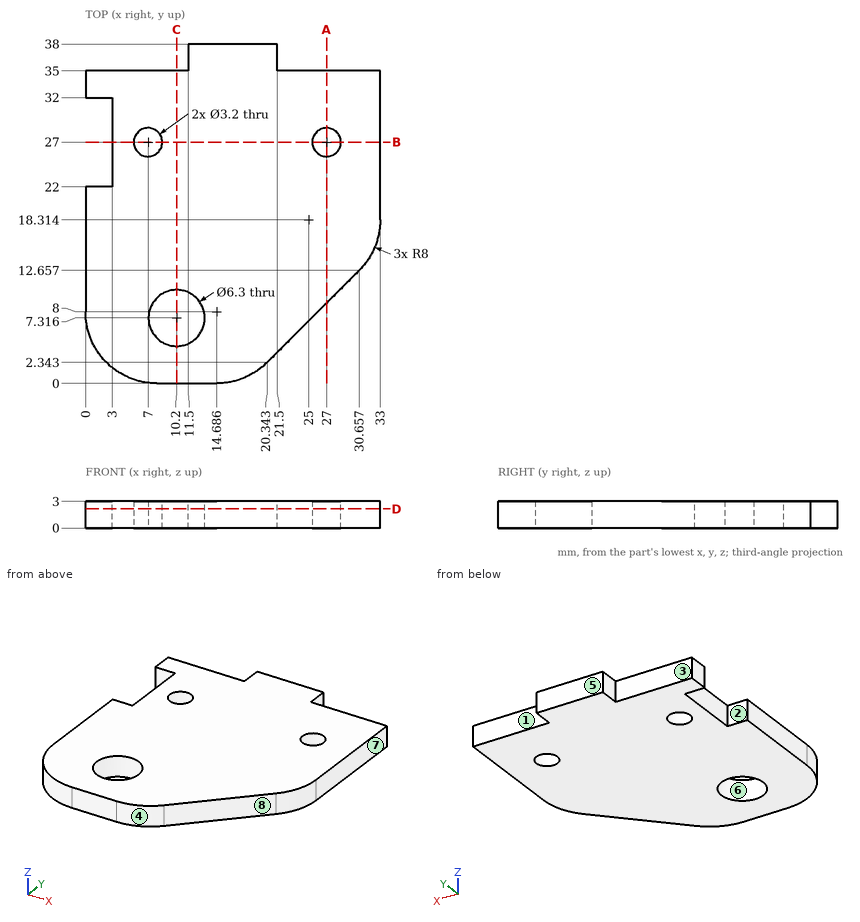
Geometry: see drawing. Coordinates: mm, zero at the bounding-box minimum. A direction names the side the tool comes from. Round coordinates to 2 decimals unless told otherwise and drop trailing zeros. Write each loop counter-clockwise with the first axis right and the second up, starting at its lowest first coordinate (ties: lowest second). Pieces come first, ordered by that corner, then holes.
1) Ray query, L1, parallel to Y at x = 10.2, z = 1.5; L2, parallel to Y at x = 21, z = 0.75; L3, parallel to Y at x = 27, z = 2.5. Return the intervals inside material, ascending.
2) Cut plane B-B (y = 27). Return the cut outline in (x, z), then the cut area to 3 significant figures.
3) Reachability of the marked faces 1, 2, 3 and 4 from +Z, -Z, +X, -X, +Y, -Y: full face, straight path, thin tool, end or side. Return the list, or none.
4) Cut plane A-A (x = 27). Return the cut outline in (y, z), then the cut area to 3 significant figures.
5) Cut plane C-C (x = 10.2). Return the cut outline in (y, z), then the cut area to 3 significant figures.
6) Draft query along Y for the marked faces 5, 6, 7 and 8. Return one class per face: pulls with the +Y half, pulls with the -Y half, needs draft (parallel to the pull), parting line crosses it, or undercut.
7) Contact query for flat-ended pins moving along their axis: P1, Ø1.5, axis at x = 1, z = 2, coming from the +Y side; P2, Ø0.9, axis at y = 37, z = 2, coming from the +X side; P3, Ø1.5, axis at x = 1, z = 2, coming from the -Y side (1 decimal). Output: stop coordinate, or through.
8) Cut plane D-D (z = 2.15). Return the cut outline in (x, y), then the cut area to 3 significant figures.
Geometry says:
1. L1: y = 0 to 4.17, 10.47 to 35
1. L2: y = 3 to 38
1. L3: y = 9 to 25.4, 28.6 to 35
2. outline: (3, 0) - (5.4, 0) - (5.4, 3) - (3, 3) - close; (8.6, 0) - (25.4, 0) - (25.4, 3) - (8.6, 3) - close; (28.6, 0) - (33, 0) - (33, 3) - (28.6, 3) - close
2. area: 70.8 mm2
3. face 1: +Z, -Z, +X, +Y
3. face 2: +Z, -Z, -X
3. face 3: +Z, -Z, -X, +Y
3. face 4: +Z, -Z, +X, -Y
4. outline: (9, 0) - (25.4, 0) - (25.4, 3) - (9, 3) - close; (28.6, 0) - (35, 0) - (35, 3) - (28.6, 3) - close
4. area: 68.4 mm2
5. outline: (0, 0) - (4.17, 0) - (4.17, 3) - (0, 3) - close; (10.47, 0) - (35, 0) - (35, 3) - (10.47, 3) - close
5. area: 86.1 mm2
6. face 5: pulls with the +Y half
6. face 6: undercut
6. face 7: needs draft
6. face 8: pulls with the -Y half
7. P1: stops at y = 35
7. P2: stops at x = 21.5
7. P3: stops at y = 3
8. outline: (0, 8) arc R8 ccw to (8, 0) - (14.69, 0) arc R8 ccw to (20.34, 2.34) - (30.66, 12.66) arc R8 ccw to (33, 18.31) - (33, 35) - (21.5, 35) - (21.5, 38) - (11.5, 38) - (11.5, 35) - (0, 35) - (0, 32) - (3, 32) - (3, 22) - (0, 22) - close; hole circle Ø3.2 at (7, 27); hole circle Ø6.3 at (10.2, 7.32); hole circle Ø3.2 at (27, 27)
8. area: 979 mm2
